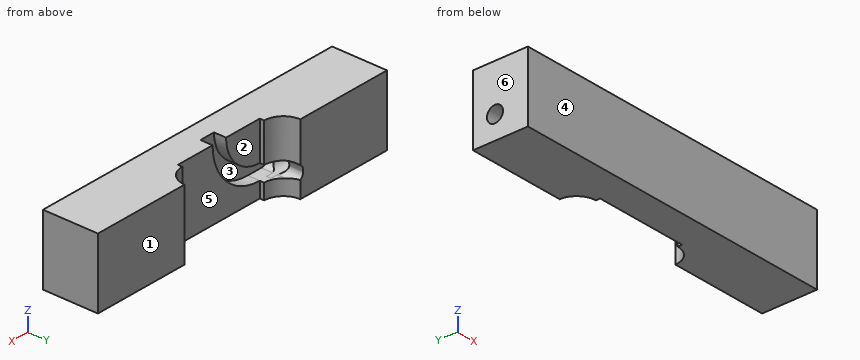
```python
from build123d import *

# Parameters (mm, degrees)
SKETCH1_W               = 38.1
SKETCH1_H               = 8.001
BOSS_EXTRUDE1_DEPTH     = 6.35
CUT_EXTRUDE1_DEPTH      = 25.4
CUT_EXTRUDE2_DEPTH      = 20.898310393
CUT_EXTRUDE2_DEPTH_BACK = 1.905
CUT_EXTRUDE3_START      = -38.1
SKETCH5_R               = 0.9271
CUT_EXTRUDE3_DEPTH      = 12.7
SKETCH6_W               = 10.795
SKETCH6_H               = 8.001
CUT_EXTRUDE4_DEPTH      = 0.508


with BuildPart() as part:
    # Sketch1 → Boss-Extrude1 (new body)
    with BuildSketch(Plane(origin=(0, 0, 0), x_dir=(1, 0, 0), z_dir=(0, 1, 0))):
        Rectangle(SKETCH1_W, SKETCH1_H)
    extrude(amount=BOSS_EXTRUDE1_DEPTH)

    # Sketch2 → Cut-Extrude1 (cut)
    with BuildSketch(Plane(origin=(0, 0, -4.0005), x_dir=(-1, 0, 0), z_dir=(0, 0, -1))):
        with BuildLine():
            Line((5.3975, 4.1275), (-5.3975, 4.1275))
            ThreePointArc((-5.3975, 4.1275), (-7.62, 6.35), (-5.3975, 8.5725))
            Line((-5.3975, 8.5725), (5.3975, 8.5725))
            ThreePointArc((5.3975, 8.5725), (7.62, 6.35), (5.3975, 4.1275))
        make_face()
    extrude(amount=-CUT_EXTRUDE1_DEPTH, mode=Mode.SUBTRACT)

    # Sketch4 → Cut-Extrude2 (cut, two sides: drawn at the far end of the back side and taken through both)
    with BuildSketch(Plane(origin=(0, 4.1275, 0), x_dir=(1, 0, 0), z_dir=(0, 1, 0)).offset(-CUT_EXTRUDE2_DEPTH_BACK)):
        with BuildLine():
            Line((0.8255, -4.0005), (-0.9525, -4.0005))
            ThreePointArc((-0.9525, -4.0005), (-2.254410358, -0.857410358), (-5.3975, 0.4445))
            Line((-5.3975, 0.4445), (-7.185501788, 0.4445))
            ThreePointArc((-7.185501788, 0.4445), (-7.769218436, 0.686283352), (-8.011001788, 1.27))
            Line((-8.011001788, 1.27), (-8.011001788, 1.397))
            ThreePointArc((-8.011001788, 1.397), (-7.769218436, 1.980716648), (-7.185501788, 2.2225))
            Line((-7.185501788, 2.2225), (-5.3975, 2.2225))
            ThreePointArc((-5.3975, 2.2225), (-0.997174501, 0.399825499), (0.8255, -4.0005))
        make_face()
    extrude(amount=CUT_EXTRUDE2_DEPTH + CUT_EXTRUDE2_DEPTH_BACK, mode=Mode.SUBTRACT)

    # Sketch5 → Cut-Extrude3 (cut)
    with BuildSketch(Plane(origin=(19.05, 0, 0), x_dir=(0, 0, -1), z_dir=(1, 0, 0)).offset(CUT_EXTRUDE3_START)):
        with Locations(Location((1.3335, 3.81, 0), (0, 0, 180))):
            Circle(SKETCH5_R)
    extrude(amount=CUT_EXTRUDE3_DEPTH, mode=Mode.SUBTRACT)

    # Sketch6 → Cut-Extrude4 (cut)
    with BuildSketch(Plane(origin=(0, 4.1275, 0), x_dir=(1, 0, 0), z_dir=(0, 1, 0))):
        Rectangle(SKETCH6_W, SKETCH6_H)
    extrude(amount=-CUT_EXTRUDE4_DEPTH, mode=Mode.SUBTRACT)


solid = part.part
```
Here's how the part is built. I have some questions about the finished solid (model axes, mm). Face numbers are marked on the shaded views. A direction names the side the tool comes from. Round coordinates to 2 decimals unless told otherwise and drop trailing zeros. Order: outer loops, then holes, each group sorted by start corner. A loop starts at its lowest first (then second) coordinate and runs counter-clockwise, first axis right, second up. Notation, with made-up numbers: M 66,-9.75 L 112,-9.75 A24 cw 112,18.25 Z; hole C 64,44.25 d1. An arc over 180 degrees is marked long. Use CSV: the item, a comma, the result in double quotes.
1) I'm going to push flat-ended pins straight in: P1, Ø1.9, axis at x = -2.5, z = 0, coming from the +Y side; P2, Ø4, axis at x = -5, z = -3, coming from the +Y side. Where does each tip first touch, or does it pass through?
Taken from the geometry:
P1,"y = 3.62"
P2,"y = 4.81"
2) If we mould it in two halves opening along X, with no side actions, what happens to the marked faces 4, 5 and 6? For each: pulls with the +X half, pulls with the -X half, needs draft (parallel to the pull), parting line crosses it, or undercut.
Taken from the geometry:
face 4,"needs draft"
face 5,"undercut"
face 6,"pulls with the -X half"
3) I need wall thicknesses on line 1 along Z through (x, y) = (-11, 3.81); line 2 along X through (y, z) = (3.75, -3); line 3 along X through (y, z) = (4.5, 3). Which ranges of each line are inside material? Lowest first, please. Write a range as [from, to].
Taken from the geometry:
line 1,"[-4, -2.26], [-0.41, 4]"
line 2,"[-19.05, -5.4], [5.4, 19.05]"
line 3,"[-19.05, -6.63], [6.63, 19.05]"
4) On a 3-axis mill with a long thin cutter (end or side, diameter ignored), from which of +Z, -Z, +X, -X, +Y, -Y can I reach the whole of each face in a straight line? I mean the marked faces 1, 2 and 3. Say none if no direction works.
Taken from the geometry:
face 1,"+Z, -Z, +X, -X, +Y"
face 2,"+Z, -Z, +Y"
face 3,"+Y"
5) I want a section at B-B (x = 2). List the corners of the cut face in (y, z) for me, then the cut area to 3 significant figures.
Taken from the geometry:
outline,"M 0,-4 L 3.62,-4 L 3.62,4 L 0,4 Z"
area,"29.0 mm^2"
